Here's how the part is built. I have some questions about the finished solid (model axes, mm). A direction names the side the tool comes from. Coordinates: 2 decimals unless noted, no trailing zeros. Write each loop counter-clockwise with the first axis right and the second up, starting at its lowest first coordinate (ties: lowest second). Pieces come first, ordered by that corner, then holes. Notation, with made-up numbers: (3, -27.75) - (52, -27.75) arc R17 cw to (52, -7.75) - close; hole circle Ø6 at (81, 34.25). An arc over 180 degrees is marked (long way). Answer in a Markdown table with one row per item. Add a question column.
Item 1: If I drill on probe 1 along Y at (x, z) = (10.5, 29); probe 2 along X at (y, z) = (19, 14), over which ranges is the centre line in solid material (lowest first)? Write a range as from..to.
Item 2: Imagine slicing it at C-C (x = -6.75). Please give me the cut outline in (y, z), plus the area to 3 significant figures.
Item 3: Imagine slicing it at D-D (y = -1). Please give me the cut outline in (x, z).
Item 4: Imagine slicing it at B-B (z = 22). Please give me the cut outline in (x, y).
Item 5: Imagine slicing it at A-A (y = 11.5). Please give me the cut outline in (x, z).
Item 6: Which directions (+Z, -Z, +X, -X, +Y, -Y) give clear straight access to the entire face, cutting with the end or side of a thin tool? Please do faces 1 (the face through (0, 19, 19)), 2 (the face through (6, 0, 19)), 3 (the face through (-12.7, 6, 19)), 4 (the face through (-6, 7, 25.4)), 5 (the face through (-6, 6, 12.7)).
Item 7: I'm going to push flat-ended pins straight in: pin 1 (4 mm diameter, centred on x = -9, y = 5, fed in from -Z); pin 2 (14 mm diameter, centred on y = 9, z = 35, fed in from -X); pin 3 (4 mm diameter, centred on y = 17, z = 17.5, fed in from +X). Where does each tip first touch, or does it pass through?
from build123d import *

# Parameters (mm, degrees)
F0_W     = 12.7
F0_H     = 38.1
F1_DEPTH = 12.7
F3_DEPTH = 12.7


with BuildPart() as f1:
    # F0 (on Right) → F1 (new body)
    with BuildSketch(Plane.YZ):
        with Locations((6.35, 19.05)):
            Rectangle(F0_W, F0_H)
    extrude(amount=F1_DEPTH)

    # F2 (on Right) → F3 (join)
    with BuildSketch(Plane.YZ):
        Polygon((-12.7, 12.7), (0, 12.7), (25.4, 12.7), (25.4, 25.4), (-12.7, 25.4), align=None)
    extrude(amount=-F3_DEPTH)


solid = f1.part
Here are the results:
| question | item | result |
|---|---|---|
| 1 | probe 1 | y = 0..12.7 |
| 1 | probe 2 | x = -12.7..0 |
| 2 | outline | (-12.7, 12.7) - (25.4, 12.7) - (25.4, 25.4) - (-12.7, 25.4) - close |
| 2 | area | 484 mm2 |
| 3 | outline | (-12.7, 12.7) - (0, 12.7) - (0, 25.4) - (-12.7, 25.4) - close |
| 4 | outline | (-12.7, -12.7) - (0, -12.7) - (0, 0) - (12.7, 0) - (12.7, 12.7) - (0, 12.7) - (0, 25.4) - (-12.7, 25.4) - close |
| 5 | outline | (-12.7, 12.7) - (0, 12.7) - (0, 0) - (12.7, 0) - (12.7, 38.1) - (0, 38.1) - (0, 25.4) - (-12.7, 25.4) - close |
| 6 | face 1 | +Z, -Z, +X, +Y |
| 6 | face 2 | +Z, -Z, +X, -Y |
| 6 | face 3 | +Z, -Z, -X, +Y, -Y |
| 6 | face 4 | +Z, -X, +Y, -Y |
| 6 | face 5 | -Z, -X, +Y, -Y |
| 7 | pin 1 | stops at z = 12.7 |
| 7 | pin 2 | stops at x = 0 |
| 7 | pin 3 | stops at x = 0 |
